Here's how the part is built. I have some questions about the finished solid (model axes, mm). Give positions to 0.01 mm unless a question says otherwise; leave off trailing zeros. Write each loop counter-clockwise with the first axis right and the second up, starting at its lowest first coordinate (ties: lowest second). Pieces come first, ordered by that corner, then holes. Notation, with made-up numbers: (38, 24.5) - (78, 24.5) arc R29 cw to (78, 45.5) - close; hole circle Ø5 at (36.25, 46). An arc over 180 degrees is marked (long way). One line per item, written item: value. Start each with the question number.
1) Imagine slicing it at B-B on z = 0. Write out the boundary of the cut face in (x, y).
2) Please list where these lines run through material, in increasing order: L1, parallel to X at y = -1.55, z = -0.5; L2, parallel to Z at x = 22.5, y = -0.25; L3, parallel to Z at x = 50, y = -0.35. Write a range as [from, to].
3) Imagine slicing it at A-A on x = -57.5. Write out the boundary of the cut face in (y, z), plus the area to 3 significant figures.
4) Imagine slicing it at D-D on z = -70. Write out the boundary of the cut face in (x, y), plus the area to 3 significant figures.
5) Imagine slicing it at C-C on y = -1. Write out the boundary of the cut face in (x, z).
6) I'm going to push a flat-ended pin straight in: P1, Ø4, axis at x = -57.5, z = -70, coming from the +Y side. Where does the tip first touch, or does it pass through?
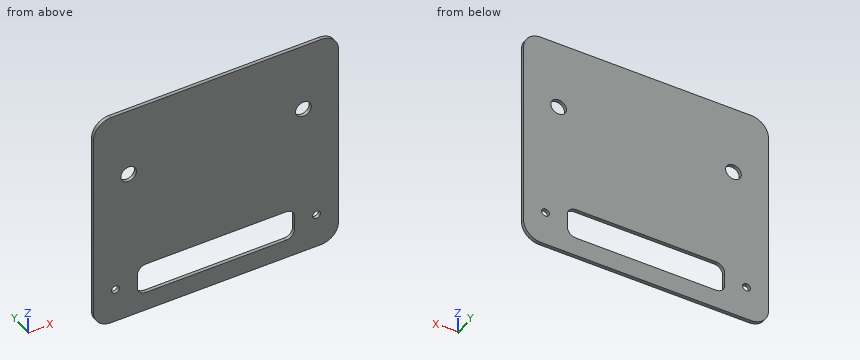
from build123d import *

# Parameters (mm, degrees)
F0_R     = 2.25
F0_R_2   = 4.5
F1_DEPTH = 2
F2_R     = 10
F3_R     = 5


with BuildPart() as f1:
    # F0 (on Front) → F1 (new body)
    with BuildSketch(Plane.XZ):
        Polygon((70, 40), (0, 40), (0, -61), (45, -61), (45, -79), (0, -79), (0, -90), (70, -90), align=None)
        with Locations((57.5, -70)):
            Circle(F0_R, mode=Mode.SUBTRACT)
        with Locations((50, 0)):
            Circle(F0_R_2, mode=Mode.SUBTRACT)
        Polygon((0, -61), (0, 40), (-70, 40), (-70, -90), (0, -90), (0, -79), (-45, -79), (-45, -61), align=None)
        with Locations((-57.5, -70)):
            Circle(F0_R, mode=Mode.SUBTRACT)
        with Locations((-50, 0)):
            Circle(F0_R_2, mode=Mode.SUBTRACT)
    extrude(amount=F1_DEPTH)

    # F2
    f2_edges = [f1.edges().sort_by_distance(p)[0] for p in [
        (70, -1, 40),
        (-70, -1, 40),
        (70, -1, -90),
        (-70, -1, -90),
    ]]
    fillet(f2_edges, radius=F2_R)

    # F3
    f3_edges = [f1.edges().sort_by_distance(p)[0] for p in [
        (45, -1, -61),
        (45, -1, -79),
        (-45, -1, -79),
        (-45, -1, -61),
    ]]
    fillet(f3_edges, radius=F3_R)


solid = f1.part
Numbers:
1. outline: (-70, -2) - (-54.5, -2) - (-54.5, 0) - (-70, 0) - close; (-45.5, -2) - (45.5, -2) - (45.5, 0) - (-45.5, 0) - close; (54.5, -2) - (70, -2) - (70, 0) - (54.5, 0) - close
2. L1: [-70, -54.47], [-45.53, 45.53], [54.47, 70]
2. L2: [-90, -79], [-61, 40]
2. L3: [-90, -4.5], [4.5, 40]
3. outline: (-2, -90) - (0, -90) - (0, -72.25) - (-2, -72.25) - close; (-2, -67.75) - (0, -67.75) - (0, 40) - (-2, 40) - close
3. area: 251 mm^2
4. outline: (-70, -2) - (-59.75, -2) - (-59.75, 0) - (-70, 0) - close; (-55.25, -2) - (-45, -2) - (-45, 0) - (-55.25, 0) - close; (45, -2) - (55.25, -2) - (55.25, 0) - (45, 0) - close; (59.75, -2) - (70, -2) - (70, 0) - (59.75, 0) - close
4. area: 82.0 mm^2
5. outline: (-70, -80) arc R10 ccw to (-60, -90) - (60, -90) arc R10 ccw to (70, -80) - (70, 30) arc R10 ccw to (60, 40) - (-60, 40) arc R10 ccw to (-70, 30) - close; hole circle Ø4.5 at (-57.5, -70); hole circle Ø9 at (-50, 0); hole (-45, -74) arc R5 ccw to (-40, -79) - (40, -79) arc R5 ccw to (45, -74) - (45, -66) arc R5 ccw to (40, -61) - (-40, -61) arc R5 ccw to (-45, -66) - close; hole circle Ø9 at (50, 0); hole circle Ø4.5 at (57.5, -70)
6. P1: through
